```python
from build123d import *

# Parameters (mm, degrees)
F0_R     = 60
F1_DEPTH = 40


with BuildPart() as f1:
    # F0 (on Front) → F1 (new body)
    with BuildSketch(Plane.XZ):
        Circle(F0_R)
    extrude(amount=F1_DEPTH)

    # F2 (on face) → F5 section 0
    with BuildSketch(Plane.XZ.offset(40), mode=Mode.PRIVATE) as f5_s0:
        Polygon((32.36068, 10.514622), (0, 34.026032), (-32.36068, 10.514622), (-20, -27.527638), (20, -27.527638), align=None)
    loft([f5_s0.sketch, Vertex(0, -120, 0)])


solid = f1.part
```
Verification items for the finished model (mm, model axes). A direction names the side the tool comes from. Coordinates: 2 decimals unless noted, no trailing zeros. Loops run counter-clockwise (first coordinate to the right, second up) from the corner with the lowest first, then second, coordinate; pieces in that order, holes last. Notation, with made-up numbers: (25, -10.75) - (31, -10.75) arc R29 cw to (31, 24.25) - close; hole circle Ø8 at (-21.75, 82.5). An arc over 180 degrees is marked (long way). Put each result on its own line as item: value.
Item 1: Section check B-B (z = -22.5). Enter the section's corners in (x, y).
Conclusion:
outline: (-55.62, -40) - (-21.63, -40) - (-16.35, -54.61) - (16.35, -54.61) - (21.63, -40) - (55.62, -40) - (55.62, 0) - (-55.62, 0) - close
Item 2: Gauge pin test, flat ends, axial feed: pin 1 Ø12 at (y, z) = (-45, 26) entering from +X; pin 2 Ø12 at (y, z) = (-99.5, -2.5) entering from -X; pin 3 Ø1.5 at (y, z) = (-54.5, 23.5) entering from -X; pin 4 Ø10 at (y, z) = (-87, 20) entering from +X. Record the tip position at first contact, or that the pin passes through.
Conclusion:
pin 1: stops at x = 55.55
pin 2: stops at x = -9.52
pin 3: stops at x = -7.12
pin 4: passes through
Item 3: Set-up check for faces 1 (the face through (26, -40, -12)), 2 (the face through (-15.902, -71.671, -4.873)): record each of +Z, -Z, +X, -X, +Y, -Y from which the full face is reachable in a straight line by a thin tool's end or side.
Conclusion:
face 1: -Y
face 2: -Z, -X, -Y
Item 4: Section check A-A (x = 23.5). Enter the section's corners in (y, z).
Conclusion:
outline: (-61.9, 7.64) - (-40, -16.76) - (-40, -55.21) - (0, -55.21) - (0, 55.21) - (-40, 55.21) - (-40, 16.95) - close
Item 5: Section check D-D (z = -5.5). Enter the section's corners in (x, y).
Conclusion:
outline: (-59.75, -40) - (-27.16, -40) - (-4, -104.02) - (4, -104.02) - (27.16, -40) - (59.75, -40) - (59.75, 0) - (-59.75, 0) - close
Item 6: Section check C-C (y = -88). Enter the section's corners in (x, z), then the cut area to 3 significant figures.
Conclusion:
outline: (-12.94, 4.21) - (-8, -11.01) - (8, -11.01) - (12.94, 4.21) - (0, 13.61) - close
area: 440 mm2
Item 7: Scan lines: line 1 along Y through (x, z) = (36, -11); line 2 along Z through (x, y) = (-2, -69); line 3 along X through (y, z) = (-83, 6). Record each from-to range of solid material in increasing order.
Conclusion:
line 1: y = -40 to 0
line 2: z = -17.55 to 20.24
line 3: x = -13.4 to 13.4
